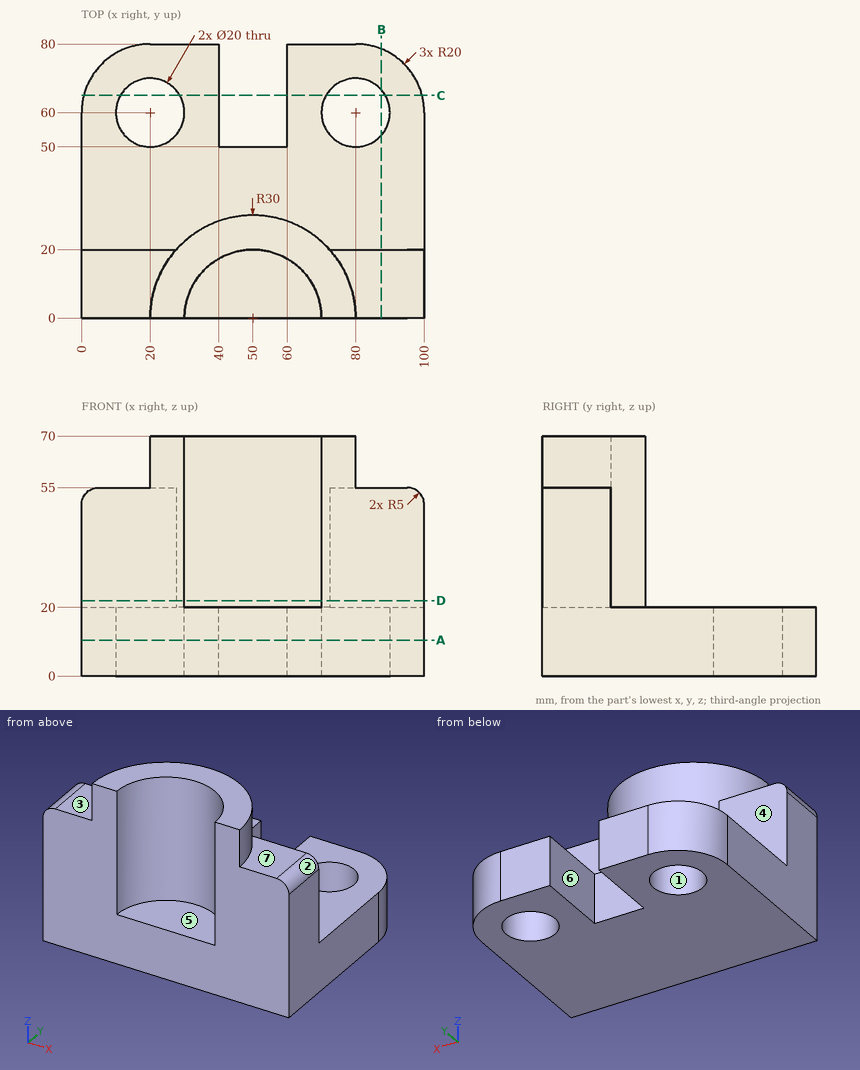
Verification items for this drawing (mm, ordinates from the low corner). A direction names the side the tool comes from. Coordinates: 2 decimals unless noted, no trailing zeros. Write each loop counter-clockwise with the first axis right and the second up, starting at its lowest first coordinate (ties: lowest second). Pieces come first, ordered by that corner, then holes. Notation, with made-up numbers: (80, 22) - (91, 22) arc R18 cw to (91, 54) - close; hole circle Ø11 at (59, 76). An arc over 180 degrees is marked (long way). One line per question, with ' | ' between items.
Item 1: Access from +Z, -Z, +X, -X, +Y, -Y to the whole of each face (thin tool, end or side, straight path). Record for the marked faces 4, 5, 6 and 7.
Determined:
face 4: +Z, -X, +Y | face 5: +Z, -Y | face 6: +Z, -Z, +Y | face 7: +Z, +X, +Y
Item 2: Gauge pin test, flat ends, axial feed: P1, Ø22, axis at x = 55, y = 5.5, coming from the +Z side; P2, Ø8.5, axis at x = 20, z = 36, coming from the +Y side; P3, Ø16, axis at y = 70, z = 10, coming from the +X side. Record the tip position at first contact, or that the pin passes through.
Determined:
P1: stops at z = 20 | P2: stops at y = 20 | P3: stops at x = 99.9
Item 3: Sectioned sample at A-A on z = 10.5. Record the boundary of the cut face in (x, y), plus the area to 3 significant figures.
Determined:
outline: (0, 0) - (100, 0) - (100, 60) arc R20 ccw to (80, 80) - (60, 80) - (60, 50) - (40, 50) - (40, 80) - (20, 80) arc R20 ccw to (0, 60) - close; hole circle Ø20 at (20, 60); hole circle Ø20 at (80, 60) | area: 6,600 mm2
Item 4: Sectioned sample at D-D on z = 22. Record the boundary of the cut face in (x, y).
Determined:
outline: (0, 0) - (30, 0) arc R20 cw to (70, 0) - (100, 0) - (100, 20) - (72.36, 20) arc R30 ccw to (27.64, 20) - (0, 20) - close
Item 5: Sectioned sample at B-B on x = 87.5. Record the boundary of the cut face in (y, z).
Determined:
outline: (0, 0) - (53.39, 0) - (53.39, 20) - (20, 20) - (20, 55) - (0, 55) - close; (66.61, 0) - (78.54, 0) - (78.54, 20) - (66.61, 20) - close
Item 6: Thickness scan on line 1 (Y direction, x = 80, z = 10); line 2 (Z direction, x = 94.5, y = 45); line 3 (Z direction, x = 85.5, y = 6). Record the ranges inside material, lowest first. Write a range as [from, to].
Determined:
line 1: y = [0, 50], [70, 80] | line 2: z = [0, 20] | line 3: z = [0, 55]
Item 7: Sectioned sample at C-C on y = 65. Record the boundary of the cut face in (x, z).
Determined:
outline: (0.64, 0) - (11.34, 0) - (11.34, 20) - (0.64, 20) - close; (28.66, 0) - (40, 0) - (40, 20) - (28.66, 20) - close; (60, 0) - (71.34, 0) - (71.34, 20) - (60, 20) - close; (88.66, 0) - (99.36, 0) - (99.36, 20) - (88.66, 20) - close
Item 8: Mould release check, pull along X, two halves, no side actions. Record for the marked faces 1, 2 and 3: pulls with the +X half, pulls with the -X half, needs draft (parallel to the pull), parting line crosses it, or undercut.
Determined:
face 1: undercut | face 2: pulls with the +X half | face 3: needs draft
